The listing builds one solid part. Answer for the finished solid, in the listing's coordinates (mm). Face numbers are marked on the shaded views. A direction names the side the tool comes from. Coordinates: 2 decimals unless noted, no trailing zeros. Write each loop counter-clockwise with the first axis right and the second up, starting at its lowest first coordinate (ties: lowest second). Pieces come first, ordered by that corner, then holes.
(1) The part is cut by section A-A on z = 254. Determine the outline of the cut face in (x, y), plus the area to 3 significant figures.
(2) Which of the six approach directions +Z, -Z, +X, -X, +Y, -Y give full straight-line access (tool end or side, diameter ignored) to the marked faces 4 and 5?
(3) The part is cut by section C-C on y = 519.5. Give the number of separate pieces and of enclosed holes in the cut face, plus the area to 3 significant figures.
(4) Given P1, Ø10, axis at x = -200.5, y = 631.5, coming from the +Z side, flat-ended and moving along its own axis, determine where the tip first touches the part or whether it passes through.
(5) For a pull along Z with two mould halves and no side action, classify the marked faces 1, 2 and 3 as +Z half, -Z half, draft (parallel to the pull), parting line (faces both ways), or undercut.
(6) Straight lines are drawn through the part: line 1 (Z direction, x = 508, y = 278); line 2 (X direction, y = 846, z = 229); line 3 (Z direction, x = -508, y = 565.5). For each, find the intervals that lie inside material, in ascending order.
(7) The part is cut by section B-B on y = 718. Determine the outline of the cut face in (x, z), plus the area to 3 significant figures.
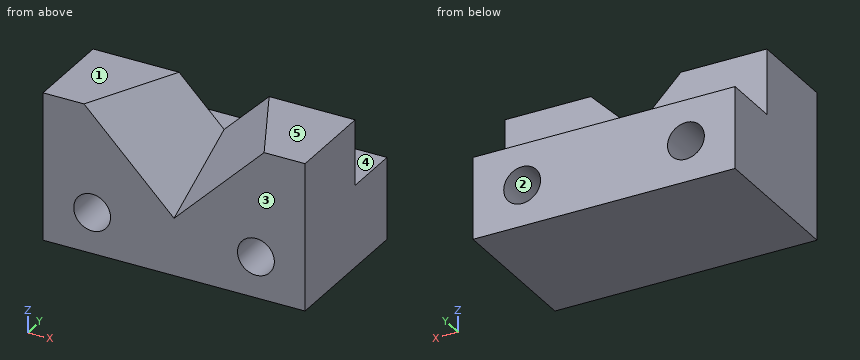
from build123d import *

# Parameters (mm, degrees)
F0_W     = 1625.6
F0_H     = 914.4
F1_DEPTH = 558.8
F2_W     = 1625.6
F2_H     = 508
F3_DEPTH = 355.6
F7_R     = 114.3
F8_DEPTH = 914.401


with BuildPart() as f1:
    # F0 (on Front) → F1 (new body)
    with BuildSketch(Plane.XZ):
        with Locations((0, 457.2)):
            Rectangle(F0_W, F0_H)
    extrude(amount=-F1_DEPTH)

    # F2 (on face) → F3 (join)
    with BuildSketch(Plane(origin=(0, 558.8, 0), x_dir=(-1, 0, 0), z_dir=(0, 1, 0))):
        with Locations((0, 254)):
            Rectangle(F2_W, F2_H)
    extrude(amount=F3_DEPTH)

    # F5 (on face) → F6 section 0
    with BuildSketch(Plane(origin=(0, 558.8, 0), x_dir=(-1, 0, 0), z_dir=(0, 1, 0))):
        Polygon((279.4, 914.4), (-279.4, 914.4), (0, 635), align=None)
    # F4 (on face) → F6 section 1
    with BuildSketch(Plane.XZ):
        Polygon((558.8, 914.4), (-558.8, 914.4), (0, 355.6), align=None)
    loft(mode=Mode.SUBTRACT)

    # F7 (on face) → F8 (cut, through all)
    with BuildSketch(Plane.XZ):
        with Locations((-508, 254)):
            Circle(F7_R)
        with Locations((508, 254)):
            Circle(F7_R)
    extrude(amount=-F8_DEPTH, mode=Mode.SUBTRACT)


solid = f1.part
Model answer:
1. outline: (-812.8, 0) - (-622.3, 0) - (-622.3, 914.4) - (-812.8, 914.4) - close; (-393.7, 0) - (393.7, 0) - (393.7, 914.4) - (-393.7, 914.4) - close; (622.3, 0) - (812.8, 0) - (812.8, 914.4) - (622.3, 914.4) - close
1. area: 1,070,000 mm2
2. face 4: +Z, +X, -X, +Y
2. face 5: +Z, +X, -X, +Y, -Y
3. separate pieces: 1
3. enclosed holes: 2
3. area: 1,310,000 mm2
4. P1: stops at z = 508
5. face 1: +Z half
5. face 2: undercut
5. face 3: draft
6. line 1: z = 0 to 139.7, 368.3 to 914.4
6. line 2: x = -812.8 to -619.53, -396.47 to 396.47, 619.53 to 812.8
6. line 3: z = 0 to 139.7, 368.3 to 508
7. outline: (-812.8, 0) - (812.8, 0) - (812.8, 508) - (-812.8, 508) - close; hole circle Ø228.6 at (-508, 254); hole circle Ø228.6 at (508, 254)
7. area: 744,000 mm2
